Check sheet for the modelled part. Datum: model origin and axes. Units: mm. Face numbers are marked on the shaded views. A direction names the side the tool comes from. Give positions to 0.01 mm unless a question says otherwise; leave off trailing zeros. Loops run counter-clockwise (first coordinate to the right, second up) from the corner with the lowest first, then second, coordinate; pieces in that order, holes last. Notation, with made-up numbers: M 75.5,78.25 L 111.5,78.25 A33 cw 111.5,111.25 Z; hole C -31.75,26 d1. An arc over 180 degrees is marked long. Write each question's results on one line, items separated by ' | '. Start each with the question number.
1. Sectioned sample at D-D on x = 36. Record the cut outline in (y, z).
2. Material ranges on line 1 along Y through (x, z) = (0, 1.5); line 2 along X through (y, z) = (-0.25, 1.45); line 3 along X through (y, z) = (-4.5, 1), recorded low to high.
3. Sectioned sample at A-A on x = 0. Record the cut outline in (y, z), and give its area (3 significant figures).
4. Tool access check on the marked faces 1, 2 and 3. Record the directions out of +Z, -Z, +X, -X, +Y, -Y that give a thin tool (end or side, any length) a straight path to the whole face; none if there is none.
5. Go/stop test with flat-tipped pins: pin 1 (3 mm diameter, centred on y = 7, z = 2.5, fed in from -X); pin 2 (2.5 mm diameter, centred on x = 36, z = 2.5, fed in from -Y); pin 3 (3 mm diameter, centred on x = 8.5, z = 2.5, fed in from +Y). Record where each tip stops, or that it passes through.
6. Sectioned sample at C-C on z = 1.7. Give the number of separate pieces and of enclosed holes in the cut face, and give its area (3 significant figures).
7. Sectioned sample at B-B on y = -7. Record the cut outline in (x, z).
```python
from build123d import *

# Parameters (mm, degrees)
SKETCH1_R           = 9.5
BOSS_EXTRUDE1_DEPTH = 5
BOSS_EXTRUDE2_DEPTH = 5
SKETCH4_R           = 0.8
CUT_EXTRUDE1_DEPTH  = 65.265761039


with BuildPart() as part:
    # Sketch1 → Boss-Extrude1 (new body)
    with BuildSketch(Plane.XY):
        Circle(SKETCH1_R)
    extrude(amount=BOSS_EXTRUDE1_DEPTH)

    # Sketch3 → Boss-Extrude2 (add)
    with BuildSketch(Plane(origin=(0, 0, 0), x_dir=(-1, 0, 0), z_dir=(0, 0, -1))):
        with BuildLine():
            Line((-8.007166595, 5.112267903), (-63.36274964, 5.112267903))
            Line((-63.36274964, 5.112267903), (-63.36274964, 0))
            Line((-63.36274964, 0), (-9.5, 0))
            ThreePointArc((-9.5, 0), (-9.119157929, 2.662885403), (-8.007166595, 5.112267903))
        make_face()
    extrude(amount=-BOSS_EXTRUDE2_DEPTH)

    # Sketch4 → Cut-Extrude1 (cut, through all)
    with BuildSketch(Plane(origin=(0, 0, 0), x_dir=(-1, 0, 0), z_dir=(0, 0, -1))):
        with Locations((0, 7)):
            Circle(SKETCH4_R)
        with Locations((4.949747468, 4.949747468)):
            Circle(SKETCH4_R)
        with Locations((7, 0)):
            Circle(SKETCH4_R)
        with Locations((4.949747468, -4.949747468)):
            Circle(SKETCH4_R)
        with Locations((0, -7)):
            Circle(SKETCH4_R)
        with Locations((-4.949747468, -4.949747468)):
            Circle(SKETCH4_R)
        with Locations((-7, 0)):
            Circle(SKETCH4_R)
        with Locations((-4.949747468, 4.949747468)):
            Circle(SKETCH4_R)
    extrude(amount=-CUT_EXTRUDE1_DEPTH, mode=Mode.SUBTRACT)


solid = part.part
```
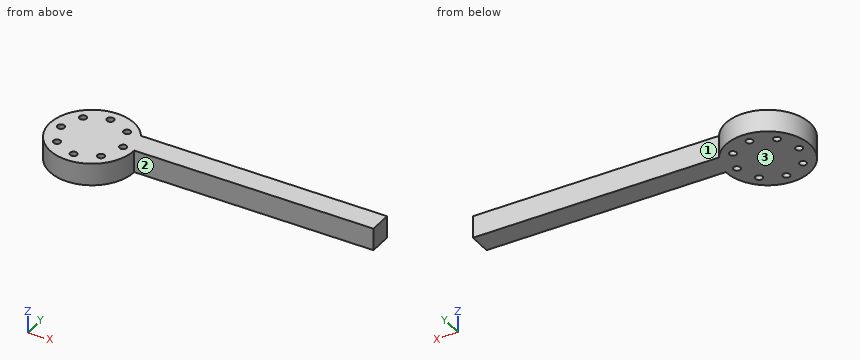
Output values:
1) outline: M 0,0 L 5.11,0 L 5.11,5 L 0,5 Z
2) line 1: -9.5 to -7.8, -6.2 to 6.2, 7.8 to 9.5 | line 2: -9.5 to -7.76, -6.24 to 6.24, 7.76 to 9.5 | line 3: -8.37 to -5.61, -4.29 to 4.29, 5.61 to 8.37
3) outline: M -9.5,0 L -7.8,0 L -7.8,5 L -9.5,5 Z; M -6.2,0 L 6.2,0 L 6.2,5 L -6.2,5 Z; M 7.8,0 L 9.5,0 L 9.5,5 L 7.8,5 Z | area: 79.0 mm2
4) face 1: +Z, -Z, +X, +Y | face 2: +Z, -Z, +X, -Y | face 3: -Z, +X, -X, +Y, -Y
5) pin 1: x = -7.75 | pin 2: y = 0 | pin 3: y = 6.42
6) separate pieces: 1 | enclosed holes: 8 | area: 545 mm2
7) outline: M -6.42,0 L -0.8,0 L -0.8,5 L -6.42,5 Z; M 0.8,0 L 6.42,0 L 6.42,5 L 0.8,5 Z
